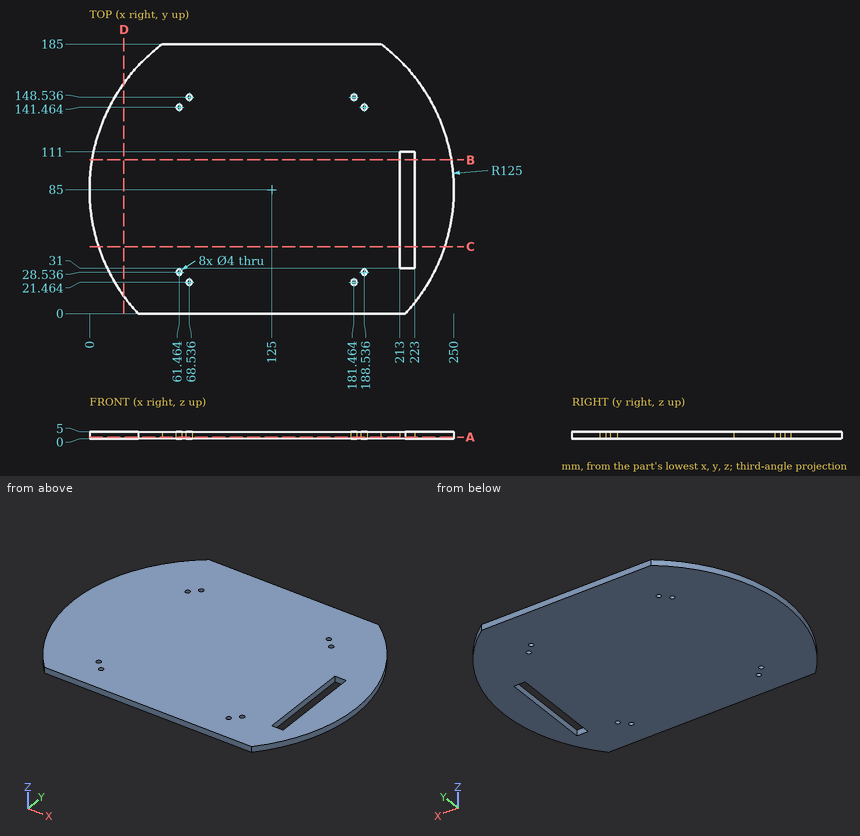
Here's the drawing with two shaded views (mm, measured from the low corner). I have some questions. Give positions to 0.01 mm unless a question says otherwise; leave off trailing zeros. Order: outer loops, then holes, each group sorted by start corner. A loop starts at its lowest first (then second) coordinate and runs counter-clockwise, first axis right, second up. Notation, with made-up numbers: M 39.25,42.5 L 95.25,42.5 A22 ccw 95.25,58.5 Z; hole C 54,-3.75 d4. An arc over 180 degrees is marked long. Answer as a JSON object with one key per item and string values. Group by question number.
1) Suppose I cut it at A-A, the plane z = 1.25. Count the separate pieces of the cut face and the enclosed holes in it, plus the area to 3 significant figures.
2) Suppose I cut it at D-D, the plane x = 23.5. Write out the boundary of the cut face in (y, z).
3) Suppose I cut it at C-C, the plane y = 46. Write out the boundary of the cut face in (x, z), plus the area to 3 significant figures.
4) Please list where these lines run through material, in increasing order: L1, parallel to X at y = 29, z = 1.95 (1 decimal); L2, parallel to X at y = 46.5, z = 4.55; L3, parallel to X at y = 101, z = 3.1. Write a range as [from, to].
5) I'm going to push flat-ended pins straight in: pin 1 Ø6.5 at (x, y) = (181.46, 148.54) entering from +Z; pin 2 Ø1.5 at (x, z) = (220.5, 3.5) entering from +Y; pin 3 Ø2 at (y, z) = (62, 1) entering from -X. Where does each tip first touch, or does it pass through?
6) Suppose I cut it at B-B, the plane y = 105.5. Write out the boundary of the cut face in (x, z), plus the area to 3 significant figures.
Results found:
{
 "1": {"separate pieces": "1", "enclosed holes": "9", "area": "40,600 mm²"},
 "2": {"outline": "M 12.04,0 L 157.96,0 L 157.96,5 L 12.04,5 Z"},
 "3": {"outline": "M 6.24,0 L 213,0 L 213,5 L 6.24,5 Z; M 223,0 L 243.76,0 L 243.76,5 L 223,5 Z", "area": "1,140 mm²"},
 "4": {"L1": "[13.2, 59.5], [63.4, 186.6], [190.5, 236.8]", "L2": "[6.08, 213], [223, 243.92]", "L3": "[1.03, 213], [223, 248.97]"},
 "5": {"pin 1": "z = 5", "pin 2": "y = 166.53", "pin 3": "x = 1.95"},
 "6": {"outline": "M 1.69,0 L 213,0 L 213,5 L 1.69,5 Z; M 223,0 L 248.31,0 L 248.31,5 L 223,5 Z", "area": "1,180 mm²"}
}
